Autodesk Fusion 360 part; units mm, degrees
sketch "Sketch1" plane through (0, 0, 0) normal (0, 0, 1) x (1, 0, 0)
  circle A0 centre (0, 0) radius 9
  circle A1 centre (0, 0) radius 22.5
  circle A2 centre (0, 0) radius 38
  dimension "d1" = 45
  dimension "d2" = 18
  dimension "d3" = 76
extrude "Extrude1" add sketch "Sketch1" along normal blind 20 contours A1
sketch "Sketch2" plane through (0, 0, 0) normal (0, 0, 1) x (1, 0, 0)
  circle A0 centre (0.2654, -30.1553) radius 2.5
  dimension "d8" = 5
extrude "Extrude4" add sketch "Sketch1" along normal blind 20 contours A1 | A2
extrude "Extrude5" cut sketch "Sketch2" along normal blind 6.312
pattern_circular "C-Pattern2" count 3 over 360 about axis through (0, 0, 20) along (0, 0, 1) of "Extrude5"
Work out the finished part from the listing and answer in its coordinate system (mm). A direction names the side the tool comes from. Coordinates: 2 decimals unless noted, no trailing zeros. Loops run counter-clockwise (first coordinate to the right, second up) from the corner with the lowest first, then second, coordinate; pieces in that order, holes last. Notation, with made-up numbers: M 56,65.25 L 79,65.25 A15 ccw 79,82.25 Z; hole C 14,82 d1. An arc over 180 degrees is marked long. Answer in a Markdown table with one row per item. Add a question column.
1. Find section D-D, the plane x = 26.5. Write down the section's boundary in (y, z).
2. Consider L1, parallel to Y at x = 0, z = 15.5; L2, parallel to Y at x = -2, z = 2.75; L3, parallel to Y at x = 8, z = 17.25. Determine where each line is inside the solid, lowest interval first.
3. Find section B-B, the plane x = -6.5. Write down the section's boundary in (y, z).
4. Flat-ended cylindrical pins translate along their axes: P1, Ø1, axis at x = -9.5, z = 15, coming from the -Y side; P2, Ø6, axis at y = -16.5, z = 8, coming from the -X side; P3, Ø2, axis at y = 20.5, z = 3.5, coming from the +X side. Find the tip coordinate at first contact, or state that the pin passes through.
5. A tool of negligible diameter and unlimited length cuts with its end or side. For faces 5 (the flat face through (8, -8, 0)), 6 (the flat face through (26, 15, 6.312)), from which of +Z, -Z, +X, -X, +Y, -Y can it reach the whole face along a straight path? Write none if from no direction.
6. Find section C-C, the plane z = 15. Write down the section's boundary in (x, y), then the cut area to 3 significant figures.
7. The mould has two halves that part along X. Classify faces 1 (the cylindrical face through (-1.172, -8.923, 9.86)), 2 (the flat face through (8, -8, 20)), 3 (the cylindrical face through (1.42, -27.94, 3.11)), 4 (the cylindrical face through (17.535, 33.713, 9.86)): pulls with the +X half, pulls with the -X half, needs draft (parallel to the pull), parting line crosses it, or undercut.
8. Find section A-A, the plane y = 0. Write down the section's boundary in (x, z).
Reported:
| question | item | result |
|---|---|---|
| 1 | outline | M -27.24,0 L 12.86,0 L 12.86,6.31 L 17.75,6.31 L 17.75,0 L 27.24,0 L 27.24,20 L -27.24,20 Z |
| 2 | L1 | y = -38 to -9, 9 to 38 |
| 2 | L2 | y = -37.95 to -31.21, -29.1 to -8.77, 8.77 to 37.95 |
| 2 | L3 | y = -37.15 to -4.12, 4.12 to 37.15 |
| 3 | outline | M -37.44,0 L -6.22,0 L -6.22,20 L -37.44,20 Z; M 6.22,0 L 37.44,0 L 37.44,20 L 6.22,20 Z |
| 4 | P1 | stops at y = -36.92 |
| 4 | P2 | stops at x = -35.52 |
| 4 | P3 | stops at x = 32.62 |
| 5 | face 5 | -Z, +X, -X, +Y, -Y |
| 5 | face 6 | -Z |
| 6 | outline | C 0,0 d76; hole C 0,0 d18 |
| 6 | area | 4,280 mm^2 |
| 7 | face 1 | undercut |
| 7 | face 2 | needs draft |
| 7 | face 3 | undercut |
| 7 | face 4 | parting line crosses it |
| 8 | outline | M -38,0 L -9,0 L -9,20 L -38,20 Z; M 9,0 L 38,0 L 38,20 L 9,20 Z |
